```python
from build123d import *

# Parameters (mm, degrees)
SKETCH1_W                                         = 80
SKETCH1_H                                         = 35
BOSS_EXTRUDE1_DEPTH                               = 5
CSK_FOR_M3_5_FLAT_HEAD_MACHINE_SCREW1_D           = 4.2
CSK_FOR_M3_5_FLAT_HEAD_MACHINE_SCREW1_CSINK_D     = 8.2
CSK_FOR_M3_5_FLAT_HEAD_MACHINE_SCREW1_CSINK_ANGLE = 90
SKETCH5_R                                         = 3.81
CUT_EXTRUDE1_DEPTH                                = 5
FILLET1_R                                         = 17.5


with BuildPart() as part:
    # Sketch1 → Boss-Extrude1 (new body)
    with BuildSketch(Plane(origin=(0, 0, 0), x_dir=(1, 0, 0), z_dir=(0, 1, 0))):
        with Locations((40, -17.5)):
            Rectangle(SKETCH1_W, SKETCH1_H)
    extrude(amount=BOSS_EXTRUDE1_DEPTH)

    # CSK for M3.5 Flat Head Machine Screw1 (through all)
    with Locations(Plane(origin=(0, 5, 0), x_dir=(1, 0, 0), z_dir=(0, 1, 0))):
        with Locations((33, -17.5), (5, -17.5)):
            CounterSinkHole(CSK_FOR_M3_5_FLAT_HEAD_MACHINE_SCREW1_D / 2, CSK_FOR_M3_5_FLAT_HEAD_MACHINE_SCREW1_CSINK_D / 2, counter_sink_angle=CSK_FOR_M3_5_FLAT_HEAD_MACHINE_SCREW1_CSINK_ANGLE)

    # Sketch5 → Cut-Extrude1 (cut)
    with BuildSketch(Plane.XZ):
        with Locations(Location((63, 17.5, 0), (0, 0, 270))):
            Circle(SKETCH5_R)
    extrude(amount=-CUT_EXTRUDE1_DEPTH, mode=Mode.SUBTRACT)

    # Fillet1
    fillet1_edges = [part.edges().sort_by_distance(p)[0] for p in [
        (80, 2.5, 35),
        (80, 2.5, 0),
    ]]
    fillet(fillet1_edges, radius=FILLET1_R - 0.0001)  # a hair under: the kernel refuses the full size


solid = part.part
```
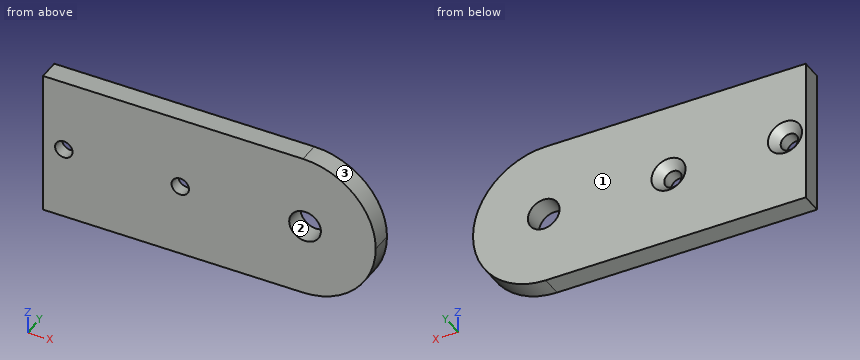
Geometry: final body of the model. Coordinates: model frame, mm. Face numbers are marked on the shaded views. Give positions to 0.01 mm unless a question says otherwise; leave off trailing zeros. Loops run counter-clockwise (first coordinate to the right, second up) from the corner with the lowest first, then second, coordinate; pieces in that order, holes last. Notation, with made-up numbers: (52, -10) -> (87, -10) arc R20 cw to (87, 15) -> close; hole circle Ø1 at (21.25, 43.5). An arc over 180 degrees is marked (long way). Use one line per item in the form item = value.
Item 1: Section query A-A on x = 33. Output: boundary loops of the cut face in (y, z), and give its area (3 significant figures).
A:
outline = (0, 0) -> (5, 0) -> (5, 13.4) -> (3, 15.4) -> (0, 15.4) -> close; (0, 19.6) -> (3, 19.6) -> (5, 21.6) -> (5, 35) -> (0, 35) -> close
area = 150 mm^2
Item 2: Section query C-C on z = 25. Output: boundary loops of the cut face in (x, y), and give its area (3 significant figures).
A:
outline = (0, 0) -> (78.31, 0) -> (78.31, 5) -> (0, 5) -> close
area = 392 mm^2
Item 3: Section query B-B on y = 3.8. Give the number of separate pieces and of enclosed holes in the cut face, and give its area (3 significant figures).
A:
separate_pieces = 1
enclosed_holes = 3
area = 2,570 mm^2
Item 4: Section query D-D on x = 70. Output: boundary loops of the cut face in (y, z), and give its area (3 significant figures).
A:
outline = (0, 1.69) -> (5, 1.69) -> (5, 33.31) -> (0, 33.31) -> close
area = 158 mm^2
Item 5: Pin query (flat end, axial travel): P1, Ø6.5, axis at x = 33, z = 17.5, coming from the +Y side; P2, Ø4.5, axis at x = 63, z = 17.5, coming from the -Y side. Return the tip coordinate at first contact, or that it passes through.
A:
P1 = 4.15
P2 = through
Item 6: Line query: probe 1 along X at (y, z) = (1.8, 17.5); probe 2 along X at (y, z) = (1.45, 17); probe 3 along Z at (x, y) = (5, 0.65). Output: solid intervals per line, ascending.
A:
probe_1 = 0 to 2.9, 7.1 to 30.9, 35.1 to 59.19, 66.81 to 80
probe_2 = 0 to 2.96, 7.04 to 30.96, 35.04 to 59.22, 66.78 to 79.99
probe_3 = 0 to 15.4, 19.6 to 35
Item 7: Draft query along Z for the marked faces 1, 2 and 3. Return one class per face: pulls with the +Z half, pulls with the -Z half, needs draft (parallel to the pull), parting line crosses it, or undercut.
A:
face_1 = needs draft
face_2 = undercut
face_3 = pulls with the +Z half
